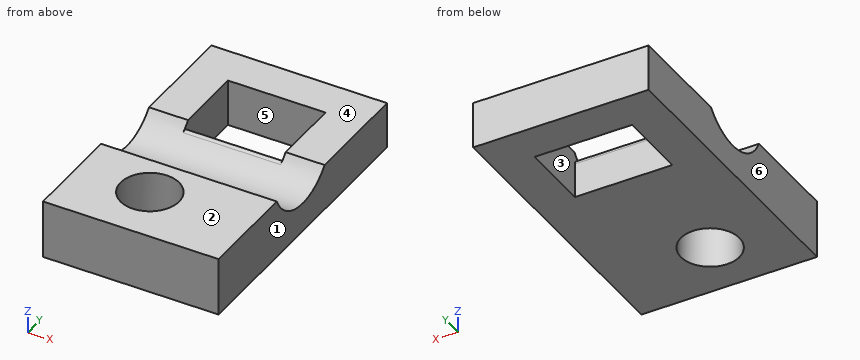
```python
from build123d import *

# Parameters (mm, degrees)
SKETCH1_W           = 18
SKETCH1_H           = 30
SKETCH1_R           = 3
SKETCH1_W_2         = 10
SKETCH1_H_2         = 7.2
BOSS_EXTRUDE1_DEPTH = 6
CUT_EXTRUDE1_DEPTH  = 19
FILLET1_R           = 0.5


with BuildPart() as part:
    # Sketch1 → Boss-Extrude1 (new body)
    with BuildSketch(Plane.XY):
        with Locations((9, 15)):
            Rectangle(SKETCH1_W, SKETCH1_H)
        with Locations((7.5, 6)):
            Circle(SKETCH1_R, mode=Mode.SUBTRACT)
        with Locations((9, 22.4)):
            Rectangle(SKETCH1_W_2, SKETCH1_H_2, mode=Mode.SUBTRACT)
    extrude(amount=BOSS_EXTRUDE1_DEPTH)

    # Sketch2 → Cut-Extrude1 (cut, through all)
    with BuildSketch(Plane(origin=(18, 0, 0), x_dir=(0, 0, -1), z_dir=(1, 0, 0))):
        with BuildLine():
            Line((-4.8, 18.888444419), (-4.8, 30))
            Line((-4.8, 30), (-6, 30))
            Line((-6, 30), (-6, 10.352419985))
            ThreePointArc((-6, 10.352419985), (-3.049660577, 14.29001992), (-4.8, 18.888444419))
        make_face()
    extrude(amount=-CUT_EXTRUDE1_DEPTH, mode=Mode.SUBTRACT)

    # Fillet1
    fillet1_edges = [part.edges().sort_by_distance(p)[0] for p in [
        (9, 18.8, 4.69852973),
    ]]
    fillet(fillet1_edges, radius=FILLET1_R)


solid = part.part
```
Source: CAD feature listing. Evaluate the final solid. Frame: model axes, mm. Face numbers are marked on the shaded views. A direction names the side the tool comes from. Give positions to 0.01 mm unless a question says otherwise; leave off trailing zeros. Order: outer loops, then holes, each group sorted by start corner. A loop starts at its lowest first (then second) coordinate and runs counter-clockwise, first axis right, second up. Notation, with made-up numbers: (-7, -16) -> (43, -16) arc R12 cw to (43, 1) -> close; hole circle Ø7 at (6.25, 87.5). An arc over 180 degrees is marked (long way). Use a Markdown table: item, result.
Q1. Section B-B (z = 2.1). Return the cut outline in (x, y).
A:
| item | result |
|---|---|
| outline | (0, 0) -> (18, 0) -> (18, 30) -> (0, 30) -> close; hole (4, 18.8) -> (14, 18.8) -> (14, 26) -> (4, 26) -> close; hole circle Ø6 at (7.5, 6) |
Q2. First-contact query: P1, Ø1, axis at y = 14.5, z = 5, coming from the -X side; P2, Ø5, axis at x = 13, y = 21, coming from the +Z side; P3, Ø2, axis at x = 9.5, y = 19, coming from the +Z side. Flat tips, straight axial feed; report the tip coordinate or a pass-through.
A:
| item | result |
|---|---|
| P1 | through |
| P2 | z = 4.8 |
| P3 | z = 4.08 |
Q3. Section A-A (y = 6). Return the cut outline in (x, z), and give its area (3 significant figures).
A:
| item | result |
|---|---|
| outline | (0, 0) -> (4.5, 0) -> (4.5, 6) -> (0, 6) -> close; (10.5, 0) -> (18, 0) -> (18, 6) -> (10.5, 6) -> close |
| area | 72.0 mm^2 |
Q4. Material intervals for line 1 (Y direction, x = 7.5, z = 2.85); line 2 (X direction, y = 22, z = 1.8); line 3 (Y direction, x = 7.5, z = 3.4), sorted ascending. Write a range as [from, to].
A:
| item | result |
|---|---|
| line 1 | [0, 3], [9, 18.8], [26, 30] |
| line 2 | [0, 4], [14, 18] |
| line 3 | [0, 3], [9, 13.02], [16.98, 18.8], [26, 30] |
Q5. Pull-direction query (X, two-part tool) for the marked faces 1, 2 and 3; classes: +X half, -X half, draft (parallel to the pull), parting line (faces both ways), or undercut.
A:
| item | result |
|---|---|
| face 1 | +X half |
| face 2 | draft |
| face 3 | undercut |
Q6. Section D-D (x = 2.75). Return the cut outline in (y, z), and give its area (3 significant figures).
A:
| item | result |
|---|---|
| outline | (0, 0) -> (30, 0) -> (30, 4.8) -> (18.89, 4.8) arc R5.1 cw to (10.35, 6) -> (0, 6) -> close |
| area | 147 mm^2 |
Q7. Access query for the marked faces 4, 5 and 6. Directions: +Z, -Z, +X, -X, +Y, -Y. A direction counts if a zero-diameter tool reaches every point of the face in a straight line with its end or side. Return the directions, or none.
A:
| item | result |
|---|---|
| face 4 | +Z, +X, -X, +Y |
| face 5 | +Z, -Z |
| face 6 | +Z, -Z, -X, +Y, -Y |
Q8. Section C-C (x = 10). Return the cut outline in (y, z), and give its area (3 significant figures).
A:
| item | result |
|---|---|
| outline | (0, 0) -> (4.34, 0) -> (4.34, 6) -> (0, 6) -> close; (7.66, 0) -> (18.8, 0) -> (18.8, 3.58) arc R0.5 ccw to (18.01, 3.98) arc R5.1 cw to (10.35, 6) -> (7.66, 6) -> close; (26, 0) -> (30, 0) -> (30, 4.8) -> (26, 4.8) -> close |
| area | 92.4 mm^2 |
